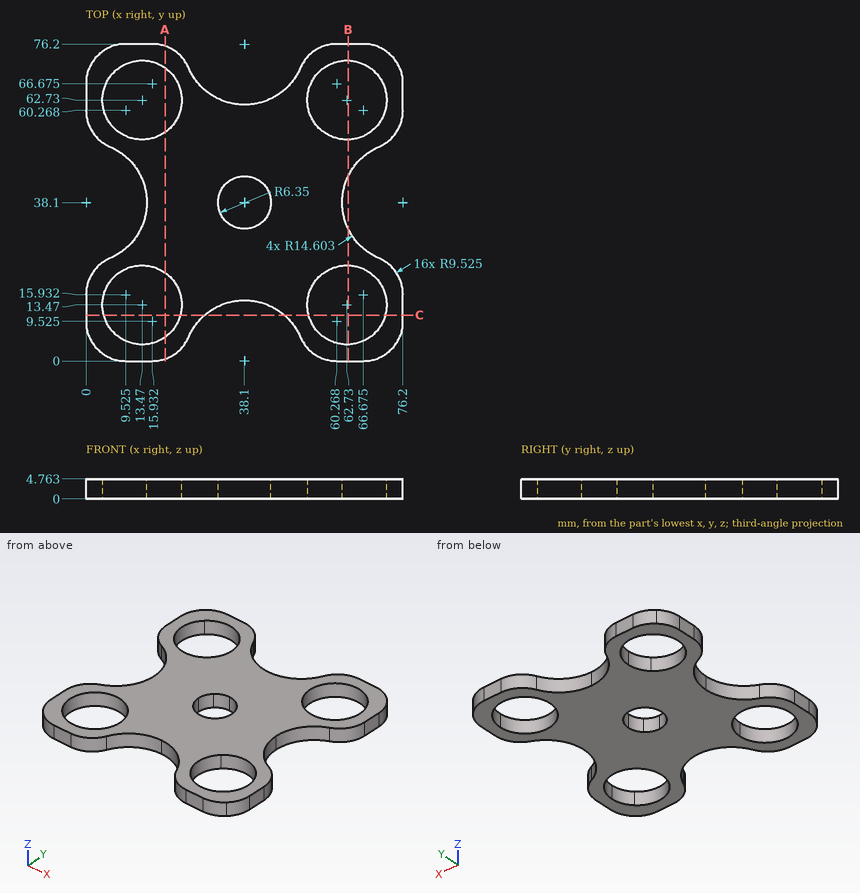
Verification items for this drawing (mm, ordinates from the low corner). Give positions to 0.01 mm unless a question says otherwise; leave off trailing zeros. Loops run counter-clockwise (first coordinate to the right, second up) from the corner with the lowest first, then second, coordinate; pieces in that order, holes last. Notation, with made-up numbers: M 7,18 L 14,18 A17 cw 14,47 Z; hole C -9,59 d8. An arc over 180 degrees is marked long. Answer as CSV lines item,"result".
Item 1: Depth check by flat-ended pin: P1, Ø1.5, axis at y = 43, z = 0.5, coming from the +X side (1 decimal). Enter the tip coordinate at first touch or a pass-through.
Values:
P1,"stops at x = 62.7"
Item 2: Cross-section at C-C on y = 11. Record the cut outline in (x, z) (1 decimal).
Values:
outline,"M 0,0 L 4.3,0 L 4.3,4.8 L 0,4.8 Z; M 22.7,0 L 28.5,0 L 28.5,4.8 L 22.7,4.8 Z; M 47.7,0 L 53.5,0 L 53.5,4.8 L 47.7,4.8 Z; M 71.9,0 L 76.2,0 L 76.2,4.8 L 71.9,4.8 Z"
Item 3: Cross-section at B-B on x = 63. Count the separate pieces of the cut face and the enclosed holes in it, and give its area (3 significant figures).
Values:
separate pieces,"4"
enclosed holes,"0"
area,"122 mm²"
Item 4: Material ranges on line 1 (X direction, y = 61, z = 4.45) (1 decimal); line 2 (X direction, y = 16, z = 3.2); line 3 (Y direction, x = 68, z = 3.9) (1 decimal), recorded low to high.
Values:
line 1,"x = 0 to 4.1, 22.8 to 53.4, 72.1 to 76.2"
line 2,"x = 0 to 4.29, 22.65 to 53.55, 71.91 to 76.2"
line 3,"y = 0.1 to 5.5, 21.4 to 26, 50.2 to 54.8, 70.7 to 76.1"
Item 5: Cross-section at A-A on x = 19. Record the cut outline in (y, z) (1 decimal).
Values:
outline,"M 0.5,0 L 5.7,0 L 5.7,4.8 L 0.5,4.8 Z; M 21.2,0 L 55,0 L 55,4.8 L 21.2,4.8 Z; M 70.5,0 L 75.7,0 L 75.7,4.8 L 70.5,4.8 Z"
